from build123d import *

# Parameters (mm, degrees)
SKETCH1_W           = 431.8
SKETCH1_H           = 609.6
BOSS_EXTRUDE1_DEPTH = 1.27
SKETCH2_R           = 14.2875
CUT_EXTRUDE1_DEPTH  = 1.27
SKETCH3_OUTSIDE_W   = 583.208
SKETCH3_OUTSIDE_H   = 761.008
CUT_EXTRUDE2_DEPTH  = 2.54


with BuildPart() as part:
    # Sketch1 → Boss-Extrude1 (new body)
    with BuildSketch(Plane.XY):
        with Locations((215.9, 304.8)):
            Rectangle(SKETCH1_W, SKETCH1_H)
    extrude(amount=BOSS_EXTRUDE1_DEPTH)

    # Sketch2 → Cut-Extrude1 (cut)
    with BuildSketch(Plane(origin=(0, 0, 0), x_dir=(-1, 0, 0), z_dir=(0, 0, -1))):
        with Locations((-82.55, 355.6)):
            Circle(SKETCH2_R)
        with Locations((-342.9, 254)):
            Circle(SKETCH2_R)
    extrude(amount=-CUT_EXTRUDE1_DEPTH, mode=Mode.SUBTRACT)

    # Sketch3 outside → Cut-Extrude2 (cut)
    with BuildSketch(Plane(origin=(0, 0, 0), x_dir=(-1, 0, 0), z_dir=(0, 0, -1))):
        with Locations((-215.9, 304.8)):
            Rectangle(SKETCH3_OUTSIDE_W, SKETCH3_OUTSIDE_H)
        with BuildLine():
            Line((-332.352291022, 194.180969832), (-300.998694729, 16.365889198))
            ThreePointArc((-300.998694729, 16.365889198), (-144.106457916, 117.227131251), (-105.987607355, 299.806202759))
            ThreePointArc((-105.987607355, 299.806202759), (-49.054456035, 305.198434711), (-22.033314292, 355.6))
            Line((-22.033314292, 355.6), (-22.033314292, 596.899879542))
            Line((-22.033314292, 596.899879542), (-82.308891716, 596.899879542))
            ThreePointArc((-82.308891716, 596.899879542), (-268.503650886, 509.375582335), (-319.513573185, 310.059304096))
            ThreePointArc((-319.513573185, 310.059304096), (-403.272414901, 260.688950139), (-332.352291022, 194.180969832))
        make_face(mode=Mode.SUBTRACT)
    extrude(amount=-CUT_EXTRUDE2_DEPTH, mode=Mode.SUBTRACT)


solid = part.part
CAD build for the part. Positions are in the model's coordinates, mm. Round coordinates to 2 decimals unless told otherwise and drop trailing zeros. Write each loop counter-clockwise with the first axis right and the second up, starting at its lowest first coordinate (ties: lowest second). Pieces come first, ordered by that corner, then holes.
(1) Slice it at D-D, the plane x = 174. Write the cut outline in (y, z), and give its area (3 significant figures).
(2) Mould opens along X. For faces 1 (the face through (49.752, 304.742, 0.626)), 2 (the face through (210, 311, 0)) say: pulls with the +X half, pulls with the -X half, needs draft (parallel to the pull), parting line crosses it, or undercut.
(3) Slice it at B-B, the plane x = 342.9. Write the cut outline in (y, z).
(4) Probe line 1 along Y through (x, z) = (342.9, 0.5); line 2 along Y through (x, z) = (82.55, 0.35); line 3 along X through (y, z) = (258.5, 1.2). List the from-to ranges inside material, lowest first.
(5) Slice it at C-C, the plane z = 1. Count the separate pieces of the cut face and the enclosed holes in it, and give its area (3 significant figures).
(6) Slice it at A-A, the plane y = 254. Write the cut outline in (x, z), and give its area (3 significant figures).
From the geometry:
1. outline: (81.67, 0) - (578.9, 0) - (578.9, 1.27) - (81.67, 1.27) - close
1. area: 631 mm2
2. face 1: undercut
2. face 2: needs draft
3. outline: (193.26, 0) - (239.71, 0) - (239.71, 1.27) - (193.26, 1.27) - close; (268.29, 0) - (314.74, 0) - (314.74, 1.27) - (268.29, 1.27) - close
4. line 1: y = 193.26 to 239.71, 268.29 to 314.74
4. line 2: y = 295.08 to 341.31, 369.89 to 596.9
4. line 3: x = 101.64 to 329.34, 356.46 to 403.47
5. separate pieces: 1
5. enclosed holes: 2
5. area: 133,000 mm2
6. outline: (101.6, 0) - (328.61, 0) - (328.61, 1.27) - (101.6, 1.27) - close; (357.19, 0) - (403.64, 0) - (403.64, 1.27) - (357.19, 1.27) - close
6. area: 347 mm2
